Geometry check sheet. Reference: the model listing, model coordinates, mm. A direction names the side the tool comes from. Coordinates: 2 decimals unless noted, no trailing zeros. Write each loop counter-clockwise with the first axis right and the second up, starting at its lowest first coordinate (ties: lowest second). Pieces come first, ordered by that corner, then holes. Notation, with made-up numbers: M -27.75,34.5 L 9.25,34.5 A9 ccw 9.25,51.5 Z; hole C -25,69 d4. An arc over 180 degrees is marked long. Put each result on its own line as item: value. Start each with the question number.
1) Cross-section at A-A on x = 25.5. Record the cut outline in (y, z).
2) Scan line: line 1 along Y through (x, z) = (31, 0). Record every from-to range of solid material in increasing order.
3) Set-up check for faces 4 (the cylindrical face through (26.95, -11.05, 11.07)), 5 (the flat face through (27, -8.5, 0)), 6 (the cylindrical face through (26.95, 11.07, 11.05)), 7 (the flat face through (8.5, -27, 0)), 8 (the cylindrical face through (11.05, -26.95, -11.07)): record each of +Z, -Z, +X, -X, +Y, -Y from which the full face is reachable in a straight line by a thin tool's end or side.
4) Mould release check, pull along Z, two halves, no side actions. Record for faces 1 (the cylindrical face through (41.85, -0.14, -11.07)), 2 (the flat face through (0, -27, 8.5)), 3 (the cylindrical face through (11.07, -26.95, 11.05)): released by +Z, released by -Z, zero draft, split by the parting line, or undercut.
5) Cross-section at D-D on y = 4.5. Record the cut outline in (x, z).
6) Gauge pin test, flat ends, axial feed: pin 1 (3 mm diameter, centred on x = 3.5, y = -30.5, fed in from +Z); pin 2 (5 mm diameter, centred on x = -3, y = -32, fed in from -Z); pin 3 (5 mm diameter, centred on x = 33, z = 3.5, fed in from -Y). Record the tip position at first contact, or that the pin passes through.
7) Cross-section at C-C on x = 3.5. Record the cut outline in (y, z).
from build123d import *

# Parameters (mm, degrees)
F0_W     = 25.4
F0_H     = 25.4
F1_DEPTH = 12.7
F2_W     = 23
F2_H     = 23
F2_W_2   = 17
F2_H_2   = 17
F3_DEPTH = 29.6
F4_R     = 1.5


# Not quite as in the source:
# - a pattern or mirror of a feature is missing from the dataset's text; its kind, count and spacing are read off the source's solid


with BuildPart() as f1:
    # F0 (on Front) → F1 (new body, symmetric)
    with BuildSketch(Plane.XZ):
        Rectangle(F0_W, F0_H)
    extrude(amount=F1_DEPTH, both=True)

    # F2 (on face) → F3 (join)
    with BuildSketch(Plane.XZ.offset(12.7)):
        Rectangle(F2_W, F2_H)
        Rectangle(F2_W_2, F2_H_2, mode=Mode.SUBTRACT)
    f3 = extrude(amount=F3_DEPTH)

    # F3_copies: F3 across plane
    add(f3.mirror(Plane(origin=(0, 0, 0), x_dir=(-0.7071067812, 0.7071067812, 0), z_dir=(0.7071067812, 0.7071067812, 0))))

    # F4
    f4_edges = [f1.edges().sort_by_distance(p)[0] for p in [
        (11.5, -27.5, 11.5),
        (11.5, -27.5, -11.5),
        (-11.5, -27.5, 11.5),
        (-11.5, -27.5, -11.5),
        (0, -42.3, 11.5),
        (11.5, -42.3, 0),
        (0, -42.3, -11.5),
        (-11.5, -42.3, 0),
        (27.5, -11.5, -11.5),
        (27.5, -11.5, 11.5),
        (42.3, -11.5, 0),
        (27.5, 11.5, -11.5),
        (42.3, 0, -11.5),
        (27.5, 11.5, 11.5),
        (42.3, 11.5, 0),
        (42.3, 0, 11.5),
    ]]
    fillet(f4_edges, radius=F4_R)


solid = f1.part
Answer key:
1. outline: M -11.5,-10 A1.5 ccw -10,-11.5 L 10,-11.5 A1.5 ccw 11.5,-10 L 11.5,10 A1.5 ccw 10,11.5 L -10,11.5 A1.5 ccw -11.5,10 Z; hole M -8.5,-8.5 L 8.5,-8.5 L 8.5,8.5 L -8.5,8.5 Z
2. line 1: y = -11.5 to -8.5, 8.5 to 11.5
3. face 4: +Z, +X, -Y
3. face 5: +X
3. face 6: +Z, +X, +Y
3. face 7: -Y
3. face 8: -Z, +X, -Y
4. face 1: released by -Z
4. face 2: undercut
4. face 3: released by +Z
5. outline: M -12.7,-12.7 L 12.7,-12.7 L 12.7,-11.5 L 40.8,-11.5 A1.5 ccw 42.3,-10 L 42.3,-8.5 L 12.7,-8.5 L 12.7,8.5 L 42.3,8.5 L 42.3,10 A1.5 ccw 40.8,11.5 L 12.7,11.5 L 12.7,12.7 L -12.7,12.7 Z
6. pin 1: stops at z = 11.5
6. pin 2: stops at z = -11.5
6. pin 3: stops at y = -11.5
7. outline: M -42.3,-10 A1.5 ccw -40.8,-11.5 L -12.7,-11.5 L -12.7,-12.7 L 12.7,-12.7 L 12.7,12.7 L -12.7,12.7 L -12.7,11.5 L -40.8,11.5 A1.5 ccw -42.3,10 L -42.3,8.5 L -12.7,8.5 L -12.7,-8.5 L -42.3,-8.5 Z
